Source: CAD feature listing. Evaluate the final solid. Frame: model axes, mm. A direction names the side the tool comes from. Coordinates: 2 decimals unless noted, no trailing zeros. Loops run counter-clockwise (first coordinate to the right, second up) from the corner with the lowest first, then second, coordinate; pieces in that order, holes last. Notation, with made-up numbers: (-26.5, 71.5) -> (32.5, 71.5) arc R16 cw to (32.5, 84.5) -> close; hole circle Ø3 at (-18.75, 59.25). An arc over 180 degrees is marked (long way). Answer as a JSON object with one key per item and string values. Group by question number.
Autodesk Inventor part; units mm, degrees
ref_plane "Work Plane1" through (0, 8.9795, -42.5) normal (0, 1, 0) x (-1, 0, 0)
ref_plane "YZ Plane" through (0, 0, 0) normal (1, 0, 0) x (0, 1, 0)
ref_plane "XY Plane" through (0, 0, 0) normal (0, 0, 1) x (1, 0, 0)
sketch "Sketch1" plane through (0, 0, 0) normal (1, 0, 0) x (0, 1, 0)
  line L0 (0, 0) -> (0, -85)
  line L1 (0, -85) -> (8, -85)
  line L2 (0, 0) -> (8, 0)
  line L3 (8, 0) -> (8, -14)
  line L4 (8, -85) -> (8, -71)
  line L5 (8, -14) -> (9, -14)
  line L6 (8, -71) -> (9, -71)
  arc A0 (10.5, -14.5) -> (10.5, -70.5) centre (267.5593, -42.5) ccw
  line L7 (8, -71) -> (10.555, -71)
  line L8 (8, -14) -> (10.555, -14)
  arc A1 (10.555, -14) -> (10.555, -71) centre (267.5473, -42.5) ccw
extrude "Extrusion1" add sketch "Sketch1" along normal mid plane 14
sketch "Sketch2" plane through (-7, 8, 0) normal (0, 1, 0) x (1, 0, 0)
  line L0 (0, 85) -> (0, 0)
  line L1 (0, 14.0338) -> (0, 5.5338)
  line L2 (14, 0) -> (14, 85)
  line L3 (14, 14.0338) -> (14, 5.5338)
  arc A0 (0, 5.5338) -> (14, 5.5338) centre (7, 7.1942) ccw
  line L4 (0, 5.5338) -> (0, 0)
  line L5 (0, 0) -> (14, 0)
  line L6 (14, 0) -> (14, 5.5338)
  point P0 (7, 0)
  dimension "d13" = 8.5
extrude "Extrusion2" cut sketch "Sketch2" against normal blind 14
sketch "Sketch3" plane through (-7, 8, -71) normal (0, 1, 0) x (1, 0, 0)
  line L0 (0, 0) -> (14, 0)
  line L1 (0, 0) -> (0, 14)
  arc A0 (14, 8.5) -> (0, 8.5) centre (7, 6.7955) ccw
  line L2 (0, 8.5) -> (0, 14)
  line L3 (0, 14) -> (14, 14)
  line L4 (14, 14) -> (14, 8.5)
  line L5 (14, -65.4662) -> (14, 14)
  line L6 (0, 14) -> (0, 8.5)
  line L7 (14, 8.5) -> (14, 14)
  line L8 (14, 14) -> (0, 14)
  line L9 (0, 8.5) -> (0, 14)
  line L10 (0, 14) -> (14, 14)
  line L11 (14, 14) -> (14, 8.5)
  line L12 (14, 14) -> (14, 0)
  arc A1 (14, 8.5) -> (0, 8.5) centre (7, 6.7955) ccw
  point P0 (7, -71)
extrude "Extrusion3" cut sketch "Sketch3" against normal blind 14 contours L1 L3 A0 | A0 L3 L4
sketch "Sketch4" plane through (-7, 8, -71) normal (0, 1, 0) x (1, 0, 0)
  arc A0 (14, 8.5) -> (0, 8.5) centre (7, 6.7955) ccw
  line L0 (7, 0.0396) -> (7, 3.0396)
  circle A1 centre (7, 9) radius 3
  point P0 (7, -71)
extrude "Extrusion4" cut sketch "Sketch4" against normal blind 14
sketch "Sketch5" plane through (-7, 8, -14) normal (0, 1, 0) x (1, 0, 0)
  circle A0 centre (7, -9) radius 3
  point P0 (7, -14)
extrude "Extrusion5" cut sketch "Sketch5" against normal blind 14
sketch "Sketch6" plane through (0, 0, -7.1942) normal (0, -1, 0) x (1, 0, 0)
  point P0 (0, 7.1942)
sketch "Sketch7" plane through (0, 0, -7.1942) normal (0, -1, 0) x (1, 0, 0)
  circle A0 centre (0, 2.1942) radius 3
  line L0 (0, -0.8058) -> (0, -3.8058)
  circle A1 centre (0, -72.8058) radius 3
  line L1 (0, -69.8058) -> (0, -66.8058)
  line L2 (0, -66.8058) -> (-5, -66.8058)
  line L3 (-5, -66.8058) -> (5, -66.8058)
  line L4 (-5, -66.8058) -> (5, -66.8058)
  line L5 (5, -66.8058) -> (5, -56.7258)
  line L6 (5, -56.7258) -> (-5, -56.7258)
  line L7 (-5, -56.7258) -> (-5, -66.8058)
  line L8 (0, -56.7258) -> (0, -56.2258)
  line L9 (-5, -56.2258) -> (5, -56.2258)
  line L10 (5, -56.2258) -> (5, -46.1458)
  line L11 (5, -46.1458) -> (-5, -46.1458)
  line L12 (-5, -46.1458) -> (-5, -56.2258)
  line L13 (0, -46.1458) -> (0, -45.6458)
  line L14 (-5, -45.6458) -> (5, -45.6458)
  line L15 (5, -45.6458) -> (5, -35.5658)
  line L16 (5, -35.5658) -> (-5, -35.5658)
  line L17 (-5, -35.5658) -> (-5, -45.6458)
  line L18 (0, -35.5658) -> (0, -35.0658)
  line L19 (-5, -35.0658) -> (5, -35.0658)
  line L20 (5, -35.0658) -> (5, -24.9858)
  line L21 (5, -24.9858) -> (-5, -24.9858)
  line L22 (-5, -24.9858) -> (-5, -35.0658)
  line L23 (0, -24.9858) -> (0, -24.4858)
  line L24 (-5, -24.4858) -> (5, -24.4858)
  line L25 (5, -24.4858) -> (5, -14.4058)
  line L26 (5, -14.4058) -> (-5, -14.4058)
  line L27 (-5, -14.4058) -> (-5, -24.4858)
  line L28 (0, -14.4058) -> (0, -13.9058)
  line L29 (-5, -13.9058) -> (5, -13.9058)
  line L30 (5, -13.9058) -> (5, -3.8058)
  line L31 (5, -3.8058) -> (-5, -3.8058)
  line L32 (-5, -3.8058) -> (-5, -13.9058)
  point P0 (0, 7.1942)
extrude "Extrusion6" cut sketch "Sketch7" against normal blind 1.5 contours L6 L5 L3 L2 L7 | L31 L30 L29 L32
sketch "Sketch8" plane through (0, 0, -7.1942) normal (0, -1, 0) x (1, 0, 0)
  line L0 (-5, -56.7258) -> (5, -56.7258)
  line L1 (0, -56.7258) -> (0, -56.2258)
  line L2 (-5, -56.2258) -> (5, -56.2258)
  line L3 (5, -56.2258) -> (5, -46.1458)
  line L4 (5, -46.1458) -> (-5, -46.1458)
  line L5 (-5, -46.1458) -> (-5, -56.2258)
  line L6 (0, -46.1458) -> (0, -45.6458)
  line L7 (-5, -45.6458) -> (5, -45.6458)
  line L8 (5, -45.6458) -> (5, -35.5658)
  line L9 (5, -35.5658) -> (-5, -35.5658)
  line L10 (-5, -35.5658) -> (-5, -45.6458)
  line L11 (0, -35.5658) -> (0, -35.0658)
  line L12 (-5, -35.0658) -> (5, -35.0658)
  line L13 (5, -35.0658) -> (5, -24.9858)
  line L14 (5, -24.9858) -> (-5, -24.9858)
  line L15 (-5, -24.9858) -> (-5, -35.0658)
  line L16 (0, -24.9858) -> (0, -24.4858)
  line L17 (-5, -24.4858) -> (5, -24.4858)
  line L18 (5, -24.4858) -> (5, -14.4058)
  line L19 (5, -14.4058) -> (-5, -14.4058)
  line L20 (-5, -14.4058) -> (-5, -24.4858)
  point P0 (0, 7.1942)
  dimension "d75" = 0.5
  dimension "d76" = 10.08
  dimension "d77" = 0.5
  dimension "d78" = 10.08
  dimension "d79" = 0.5
  dimension "d80" = 10.08
  dimension "d81" = 0.5
  dimension "d82" = 10.08
extrude "Extrusion7" cut sketch "Sketch8" against normal blind 1
sketch "Sketch9" plane through (0, 1.5, -7.1942) normal (0, -1, 0) x (1, 0, 0)
  line L0 (-5, -66.8058) -> (-5, -56.7258)
  line L1 (5, -56.7258) -> (5, -66.8058)
  line L2 (-5, -59.2658) -> (5, -59.2658)
  line L3 (-5, -64.2658) -> (5, -64.2658)
  line L4 (-5, -64.2658) -> (-5, -59.2658)
  line L5 (5, -64.2658) -> (5, -59.2658)
  line L6 (5, -64.2658) -> (5, -59.2658)
  point P0 (0, 7.1942)
extrude "Extrusion8" cut sketch "Sketch9" against normal blind 20
sketch "Sketch10" plane through (0, 1, -7.1942) normal (0, -1, 0) x (1, 0, 0)
  line L0 (-5, -56.2258) -> (-5, -46.1458)
  line L1 (5, -46.1458) -> (5, -56.2258)
  line L2 (-5, -53.6858) -> (5, -53.6858)
  line L3 (-5, -48.6858) -> (5, -48.6858)
  line L4 (5, -48.6858) -> (5, -53.6858)
  line L5 (-5, -48.6858) -> (-5, -53.6858)
  point P0 (0, 7.1942)
  dimension "d95" = 20
  dimension "d96" = 0
extrude "Extrusion9" cut sketch "Sketch10" against normal blind 20
sketch "Sketch11" plane through (0, 1, -7.1942) normal (0, -1, 0) x (1, 0, 0)
  line L0 (-5, -45.6458) -> (-5, -35.5658)
  line L1 (5, -35.5658) -> (5, -45.6458)
  line L2 (-5, -43.1058) -> (5, -43.1058)
  line L3 (-5, -38.1058) -> (5, -38.1058)
  line L4 (5, -38.1058) -> (5, -43.1058)
  line L5 (-5, -38.1058) -> (-5, -43.1058)
  point P0 (0, 7.1942)
extrude "Extrusion10" cut sketch "Sketch11" against normal blind 20
sketch "Sketch12" plane through (0, 1, -7.1942) normal (0, -1, 0) x (1, 0, 0)
  line L0 (-5, -35.0658) -> (-5, -24.9858)
  line L1 (5, -24.9858) -> (5, -35.0658)
  line L2 (-5, -32.5258) -> (5, -32.5258)
  line L3 (-5, -27.5258) -> (5, -27.5258)
  line L4 (5, -27.5258) -> (5, -32.5258)
  line L5 (-5, -27.5258) -> (-5, -32.5258)
  point P0 (0, 7.1942)
extrude "Extrusion11" cut sketch "Sketch12" against normal blind 20
sketch "Sketch13" plane through (0, 1, -7.1942) normal (0, -1, 0) x (1, 0, 0)
  line L0 (-5, -24.4858) -> (-5, -14.4058)
  line L1 (-5, -21.9458) -> (5, -21.9458)
  line L2 (-5, -16.9458) -> (5, -16.9458)
  line L3 (5, -16.9458) -> (5, -21.9458)
  line L4 (5, -14.4058) -> (5, -24.4858)
  line L5 (-5, -16.9458) -> (-5, -21.9458)
  point P0 (0, 7.1942)
extrude "Extrusion12" cut sketch "Sketch13" against normal blind 20
sketch "Sketch14" plane through (0, 1.5, -7.1942) normal (0, -1, 0) x (1, 0, 0)
  line L0 (-5, -13.9058) -> (-5, -3.8058)
  line L1 (5, -3.8058) -> (5, -13.9058)
  line L2 (-5, -11.3558) -> (5, -11.3558)
  line L3 (-5, -6.3558) -> (5, -6.3558)
  line L4 (5, -6.3558) -> (5, -11.3558)
  line L5 (-5, -6.772) -> (-5, -11.3558)
  line L6 (-5, -6.3558) -> (-5, -11.3558)
  point P0 (0, 7.1942)
extrude "Extrusion13" cut sketch "Sketch14" against normal blind 20
sketch "Sketch15" plane through (0, 1.5, -7.1942) normal (0, -1, 0) x (1, 0, 0)
  point P0 (0, 7.1942)
sketch "Sketch16" plane through (0, 1.5, -7.1942) normal (0, -1, 0) x (1, 0, 0)
  point P0 (0, 7.1942)
sketch "Sketch17" plane through (0, 0, -7.1942) normal (0, -1, 0) x (1, 0, 0)
  point P0 (0, 7.1942)
sketch "Sketch18" plane through (7, 0, 0) normal (1, 0, 0) x (0, 0, -1)
  point P0 (0, 0)
sketch "Sketch19" plane through (0, 1, -7.1942) normal (0, -1, 0) x (1, 0, 0)
  line L0 (-5, -13.9058) -> (-5, -11.3558)
  line L1 (-5, -11.3558) -> (-5, -59.3271)
  line L2 (-5, -66.8058) -> (-5, -56.7258)
  point P0 (0, 7.1942)
ref_plane "Work Plane1" through (0, 8.9795, -42.5) normal (0, 1, 0) x (-1, 0, 0)
sketch "Sketch20" plane through (0, 8.9795, -42.5) normal (0, 1, 0) x (-1, 0, 0)
  point P0 (0, 42.5)
sketch "Sketch21" plane through (-5, 0, -21.6) normal (1, 0, 0) x (0, 0, -1)
  point P0 (-21.6, 0)
properties part number "segurador das cordas" material "Steel"
1. Section query A-A on y = 7.25. State how many separate pieces and enclosed holes the cut face has, then the cut area to 3 significant figures.
2. Reachability of faces 1 (the face through (0, 5, -50.3)), 2 (the face through (-0.1, 8.98, -42.89)), 3 (the face through (0, 1.5, -73)) from +Z, -Z, +X, -X, +Y, -Y: full face, straight path, thin tool, end or side. Return the list, or none.
3. Ray query, L1, parallel to X at y = 8, z = -68.5; L2, parallel to X at y = 4.75, z = -78; L3, parallel to Y at x = -2.75, z = -40. Return the intervals inside material, ascending.
4. Section query B-B on z = -68.5. Return loops of the section in (x, y).
5. Mould query, pull axis Z, two halves, no side actions, for faces 4 (the face through (0, 5, -45.3)), 5 (the face through (-0.1, 8, -76.5)), 6 (the face through (-6, 9, -14)). Classes: pulls with the +Z half, pulls with the -Z half, needs draft (parallel to the pull), parting line crosses it, or undercut.
6. Section query D-D on x = 5.75. Return loops of the section in (y, z) (1 decimal).
7. Pin query (flat end, axial travel): pin 1 Ø1.1 at (x, y) = (1.5, 0.5) entering from -Z; pin 2 Ø0.8 at (x, z) = (0.5, -22.5) entering from -Y; pin 3 Ø4 at (x, z) = (-2.5, -5.5) entering from +Y. Return the tip coordinate at first contact, or that it passes through.
Solved:
{
 "1": {"separate pieces": "1", "enclosed holes": "8", "area": "794 mm^2"},
 "2": {"face 1": "+Y, -Y", "face 2": "+X, -X, +Y", "face 3": "-Y"},
 "3": {"L1": "-7 to -5, 5 to 7", "L2": "-7 to -2.24, 2.24 to 7", "L3": "1 to 8.99"},
 "4": {"outline": "(-7, 0) -> (-5, 0) -> (-5, 10.29) -> (-7, 10.29) -> close; (5, 0) -> (7, 0) -> (7, 10.29) -> (5, 10.29) -> close"},
 "5": {"face 4": "undercut", "face 5": "needs draft", "face 6": "pulls with the +Z half"},
 "6": {"outline": "(0, -82.1) -> (8, -82.1) -> (8, -71) -> (10.6, -71) arc R258.6 cw to (10.5, -70.5) arc R258.6 cw to (10.5, -14.5) arc R258.6 cw to (10.6, -14) -> (8, -14) -> (8, -2.9) -> (0, -2.9) -> close"},
 "7": {"pin 1": "z = -84.94", "pin 2": "y = 1", "pin 3": "y = 8"}
}
